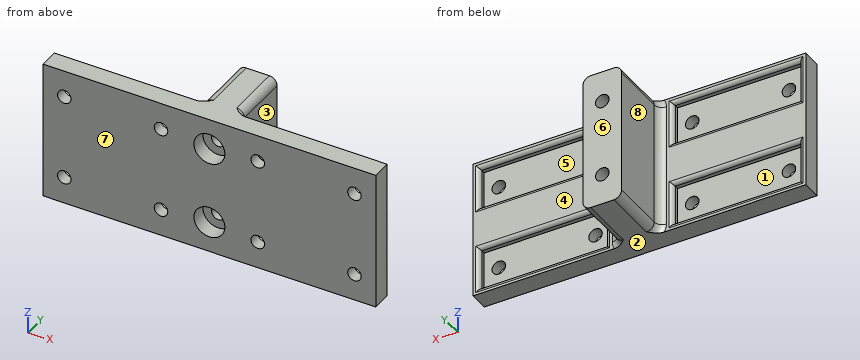
```python
from build123d import *

# Parameters (mm, degrees)
SKETCH_1_W          = 86
SKETCH_1_H          = 36
EXTRUDE_1_DEPTH     = 5
SKETCH_5_W          = 32.6
SKETCH_5_H          = 10.6
SKETCH_5_R          = 1.75
CUT_EXTRUDE_2_DEPTH = 2
SKETCH_5_3_R        = 1.75
CUT_EXTRUDE_3_DEPTH = 47.882832679
FILLET_2_R          = 1
SKETCH_8_W          = 10
SKETCH_8_H          = 36
EXTRUDE_2_DEPTH     = 16.5
SKETCH_9_R          = 1.75
CUT_EXTRUDE_4_DEPTH = 52.334686129
FILLET_3_R          = 2
FILLET_4_R          = 2
SKETCH_10_R         = 4
CUT_EXTRUDE_5_DEPTH = 4


with BuildPart() as part:
    # ｽｹｯﾁ1 → ﾎﾞｽ - 押し出し1 (new body)
    with BuildSketch(Plane(origin=(0, 0, 0), x_dir=(1, 0, 0), z_dir=(0, 1, 0))):
        Rectangle(SKETCH_1_W, SKETCH_1_H)
    extrude(amount=EXTRUDE_1_DEPTH)

    # ｽｹｯﾁ5 → ｶｯﾄ - 押し出し2 (cut)
    # profile 1 of 4: a face of its own
    with BuildSketch(Plane(origin=(0, 5, 0), x_dir=(1, 0, 0), z_dir=(0, 1, 0))):
        with Locations((-25, -11)):
            Rectangle(SKETCH_5_W, SKETCH_5_H)
        with Locations(Location((-37.5, -11, 0), (0, 0, 270))):
            Circle(SKETCH_5_R, mode=Mode.SUBTRACT)
        with Locations(Location((-12.5, -11, 0), (0, 0, 90))):
            Circle(SKETCH_5_R, mode=Mode.SUBTRACT)
    # profile 2 of 4: a face of its own
    with BuildSketch(Plane(origin=(0, 5, 0), x_dir=(1, 0, 0), z_dir=(0, 1, 0))):
        with Locations((-25, 11)):
            Rectangle(SKETCH_5_W, SKETCH_5_H)
        with Locations(Location((-12.5, 11, 0), (0, 0, 270))):
            Circle(SKETCH_5_R, mode=Mode.SUBTRACT)
        with Locations(Location((-37.5, 11, 0), (0, 0, 90))):
            Circle(SKETCH_5_R, mode=Mode.SUBTRACT)
    # profile 3 of 4: a face of its own
    with BuildSketch(Plane(origin=(0, 5, 0), x_dir=(1, 0, 0), z_dir=(0, 1, 0))):
        with Locations((25, 11)):
            Rectangle(SKETCH_5_W, SKETCH_5_H)
        with Locations(Location((37.5, 11, 0), (0, 0, 270))):
            Circle(SKETCH_5_R, mode=Mode.SUBTRACT)
        with Locations(Location((12.5, 11, 0), (0, 0, 90))):
            Circle(SKETCH_5_R, mode=Mode.SUBTRACT)
    # profile 4 of 4: a face of its own
    with BuildSketch(Plane(origin=(0, 5, 0), x_dir=(1, 0, 0), z_dir=(0, 1, 0))):
        with Locations((25, -11)):
            Rectangle(SKETCH_5_W, SKETCH_5_H)
        with Locations(Location((12.5, -11, 0), (0, 0, 270))):
            Circle(SKETCH_5_R, mode=Mode.SUBTRACT)
        with Locations(Location((37.5, -11, 0), (0, 0, 90))):
            Circle(SKETCH_5_R, mode=Mode.SUBTRACT)
    extrude(amount=-CUT_EXTRUDE_2_DEPTH, mode=Mode.SUBTRACT)

    # ｽｹｯﾁ5<3> → ｶｯﾄ - 押し出し3 (cut, through all)
    with BuildSketch(Plane(origin=(0, 5, 0), x_dir=(1, 0, 0), z_dir=(0, 1, 0))):
        with Locations(Location((37.5, -11, 0), (0, 0, 270))):
            Circle(SKETCH_5_3_R)
        with Locations(Location((12.5, -11, 0), (0, 0, 270))):
            Circle(SKETCH_5_3_R)
        with Locations(Location((37.5, 11, 0), (0, 0, 270))):
            Circle(SKETCH_5_3_R)
        with Locations(Location((12.5, 11, 0), (0, 0, 270))):
            Circle(SKETCH_5_3_R)
        with Locations(Location((-12.5, 11, 0), (0, 0, 270))):
            Circle(SKETCH_5_3_R)
        with Locations(Location((-12.5, -11, 0), (0, 0, 270))):
            Circle(SKETCH_5_3_R)
        with Locations(Location((-37.5, -11, 0), (0, 0, 270))):
            Circle(SKETCH_5_3_R)
        with Locations(Location((-37.5, 11, 0), (0, 0, 270))):
            Circle(SKETCH_5_3_R)
    extrude(amount=-CUT_EXTRUDE_3_DEPTH, mode=Mode.SUBTRACT)

    # ﾌｨﾚｯﾄ2
    fillet_2_edges = [part.edges().sort_by_distance(p)[0] for p in [
        (-8.7, 5, 11),
        (-25, 5, 5.7),
        (-41.3, 5, 11),
        (-25, 5, 16.3),
        (-25, 5, -16.3),
        (-41.3, 5, -11),
        (-25, 5, -5.7),
        (-8.7, 5, -11),
        (8.7, 5, -11),
        (25, 5, -5.7),
        (41.3, 5, -11),
        (25, 5, -16.3),
        (25, 5, 16.3),
        (41.3, 5, 11),
        (25, 5, 5.7),
        (8.7, 5, 11),
    ]]
    fillet(fillet_2_edges, radius=FILLET_2_R)

    # ｽｹｯﾁ8 → ﾎﾞｽ - 押し出し2 (add)
    with BuildSketch(Plane(origin=(0, 5, 0), x_dir=(1, 0, 0), z_dir=(0, 1, 0))):
        Rectangle(SKETCH_8_W, SKETCH_8_H)
    extrude(amount=EXTRUDE_2_DEPTH)

    # ｽｹｯﾁ9 → ｶｯﾄ - 押し出し4 (cut, through all)
    with BuildSketch(Plane(origin=(0, 21.5, 0), x_dir=(1, 0, 0), z_dir=(0, 1, 0))):
        with Locations(Location((0, -10, 0), (0, 0, 270))):
            Circle(SKETCH_9_R)
        with Locations(Location((0, 10, 0), (0, 0, 270))):
            Circle(SKETCH_9_R)
    extrude(amount=-CUT_EXTRUDE_4_DEPTH, mode=Mode.SUBTRACT)

    # ﾌｨﾚｯﾄ3
    fillet_3_edges = [part.edges().sort_by_distance(p)[0] for p in [
        (-5, 13.25, -18),
        (-5, 13.25, 18),
        (5, 13.25, 18),
        (5, 13.25, -18),
    ]]
    fillet(fillet_3_edges, radius=FILLET_3_R)

    # ﾌｨﾚｯﾄ4
    # the kernel refuses this fillet: 2 mm, written as the material it adds along each edge
    with BuildSketch(Plane(origin=(5, 5, 16), x_dir=(1, 0, 0), z_dir=(0, 0, -1)), Plane(origin=(-5, 5, -16), x_dir=(-1, 0, 0), z_dir=(0, 0, 1))) as fillet_4_piece_1:
        with BuildLine():
            CenterArc((FILLET_4_R, -FILLET_4_R), FILLET_4_R, 90, 90)
            Line((0, -FILLET_4_R), (0, 0))
            Line((0, 0), (FILLET_4_R, 0))
        make_face()
    extrude(amount=32)
    with BuildSketch(Plane(origin=(3, 5, 16), x_dir=(-0.5976672776328272, 0, -0.8017442392976484), z_dir=(0.8017442392976484, 0, -0.5976672776328272))) as fillet_4_piece_2_section:
        with BuildLine():
            CenterArc((2 + FILLET_4_R, FILLET_4_R), FILLET_4_R, 180, 90)
            Line((2 + FILLET_4_R, 0), (2, 0))
            Line((2, 0), (2, FILLET_4_R))
        make_face()
    fillet_4_piece_2 = revolve(axis=Axis((3, 5, 16), (0, 1, 0)), revolution_arc=233.296989237, mode=Mode.PRIVATE)
    fillet_4_piece_2 = split(fillet_4_piece_2, bisect_by=Plane(origin=(4.499877774, 5.623256904, 18), z_dir=(0, 0, -1)), keep=Keep.TOP, mode=Mode.PRIVATE)
    add(fillet_4_piece_2)
    with BuildSketch(Plane(origin=(-3, 5, 16), x_dir=(0.5976672776328272, 0, -0.8017442392976484), z_dir=(-0.8017442392976484, 0, -0.5976672776328272))) as fillet_4_piece_3_section:
        with BuildLine():
            CenterArc((2 + FILLET_4_R, -FILLET_4_R), FILLET_4_R, 90, 90)
            Line((2, -FILLET_4_R), (2, 0))
            Line((2, 0), (2 + FILLET_4_R, 0))
        make_face()
    fillet_4_piece_3 = revolve(axis=Axis((-3, 5, 16), (0, -1, 0)), revolution_arc=233.296989237, mode=Mode.PRIVATE)
    fillet_4_piece_3 = split(fillet_4_piece_3, bisect_by=Plane(origin=(-4.499877889, 5.623256622, 18), z_dir=(0, 0, -1)), keep=Keep.TOP, mode=Mode.PRIVATE)
    add(fillet_4_piece_3)
    with BuildSketch(Plane(origin=(-3, 5, -16), x_dir=(-1, 0, 0), z_dir=(0, 0, 1))) as fillet_4_piece_4_section:
        with BuildLine():
            CenterArc((2 + FILLET_4_R, -FILLET_4_R), FILLET_4_R, 90, 90)
            Line((2, -FILLET_4_R), (2, 0))
            Line((2, 0), (2 + FILLET_4_R, 0))
        make_face()
    fillet_4_piece_4 = revolve(axis=Axis((-3, 5, -16), (0, -1, 0)), revolution_arc=233.296989237, mode=Mode.PRIVATE)
    fillet_4_piece_4 = split(fillet_4_piece_4, bisect_by=Plane(origin=(-5.439550498, 5.334600403, -18), z_dir=(0, 0, 1)), keep=Keep.TOP, mode=Mode.PRIVATE)
    add(fillet_4_piece_4)
    with BuildSketch(Plane(origin=(3, 5, -16), x_dir=(-0.5976672776328279, 0, 0.8017442392976479), z_dir=(0.8017442392976479, 0, 0.5976672776328279))) as fillet_4_piece_5_section:
        with BuildLine():
            CenterArc((2 + FILLET_4_R, -FILLET_4_R), FILLET_4_R, 90, 90)
            Line((2, -FILLET_4_R), (2, 0))
            Line((2, 0), (2 + FILLET_4_R, 0))
        make_face()
    fillet_4_piece_5 = revolve(axis=Axis((3, 5, -16), (0, -1, 0)), revolution_arc=233.296989237, mode=Mode.PRIVATE)
    fillet_4_piece_5 = split(fillet_4_piece_5, bisect_by=Plane(origin=(4.499877909, 5.62325654, -18), z_dir=(0, 0, 1)), keep=Keep.TOP, mode=Mode.PRIVATE)
    add(fillet_4_piece_5)

    # ｽｹｯﾁ10 → ｶｯﾄ - 押し出し5 (cut)
    with BuildSketch(Plane(origin=(0, 0, 0), x_dir=(-1, 0, 0), z_dir=(0, -1, 0))):
        with Locations(Location((0, -10, 0), (0, 0, 90))):
            Circle(SKETCH_10_R)
        with Locations(Location((0, 10, 0), (0, 0, 90))):
            Circle(SKETCH_10_R)
    extrude(amount=-CUT_EXTRUDE_5_DEPTH, mode=Mode.SUBTRACT)


solid = part.part
```
Can you work these out from the model? Positions are in its coordinate system, mm. Face numbers are marked on the shaded views. A direction names the side the tool comes from. Round coordinates to 2 decimals unless told otherwise and drop trailing zeros. Loops run counter-clockwise (first coordinate to the right, second up) from the corner with the lowest first, then second, coordinate; pieces in that order, holes last. Notation, with made-up numbers: (50.25, 85.25) -> (68.25, 85.25) arc R18 cw to (68.25, 97.25) -> close; hole circle Ø7 at (23, 61.25). An arc over 180 degrees is marked (long way). Answer in a Markdown table with one row per item.
Item 1: If I drill on probe 1 along Z at (x, y) = (38.5, 3.5); probe 2 along X at (y, z) = (1, -11); probe 3 along X at (y, z) = (13.5, -6.5), over which ranges is the centre line in solid material (lowest first)?
Answer block:
| item | result |
|---|---|
| probe 1 | -18 to -16.3, -5.7 to 5.7, 16.3 to 18 |
| probe 2 | -43 to -39.25, -35.75 to -14.25, -10.75 to -3.87, 3.87 to 10.75, 14.25 to 35.75, 39.25 to 43 |
| probe 3 | -5 to 5 |
Item 2: Suppose I cut it at A-A, the plane x = -12.5. List the corners of the cut face in (y, z) for me, plus the area to 3 significant figures.
Answer block:
| item | result |
|---|---|
| outline | (0, -18) -> (5, -18) -> (5, -17.3) arc R1 ccw to (4, -16.3) -> (3, -16.3) -> (3, -12.75) -> (0, -12.75) -> close; (0, -9.25) -> (3, -9.25) -> (3, -5.7) -> (4, -5.7) arc R1 ccw to (5, -4.7) -> (5, 4.7) arc R1 ccw to (4, 5.7) -> (3, 5.7) -> (3, 9.25) -> (0, 9.25) -> close; (0, 12.75) -> (3, 12.75) -> (3, 16.3) -> (4, 16.3) arc R1 ccw to (5, 17.3) -> (5, 18) -> (0, 18) -> close |
| area | 116 mm² |
Item 3: Suppose I cut it at B-B, the plane y = 10.75. List the corners of the cut face in (x, z) for me.
Answer block:
| item | result |
|---|---|
| outline | (-5, -16) arc R2 ccw to (-3, -18) -> (3, -18) arc R2 ccw to (5, -16) -> (5, 16) arc R2 ccw to (3, 18) -> (-3, 18) arc R2 ccw to (-5, 16) -> close; hole circle Ø3.5 at (0, -10); hole circle Ø3.5 at (0, 10) |
Item 4: Suppose I cut it at D-D, the plane z = 10.5. Give the number of separate pieces and of enclosed holes in the cut face, plus the area to 3 significant figures.
Answer block:
| item | result |
|---|---|
| separate pieces | 6 |
| enclosed holes | 0 |
| area | 335 mm² |
Item 5: We'd pull the mould along Z, two halves only. Please class the marked faces 1, 2 and 3: released by +Z, released by -Z, zero draft, split by the parting line, or undercut.
Answer block:
| item | result |
|---|---|
| face 1 | undercut |
| face 2 | released by -Z |
| face 3 | zero draft |
Item 6: Will these pins go through, and if not, where does the flat tip stop? P1, Ø5, axis at x = 6, y = 12, coming from the -Z side; P2, Ø3, axis at x = -12.5, z = -11, coming from the +Y side; P3, Ø7, axis at y = 17, z = 0, coming from the +X side; P4, Ø5.5, axis at x = 29.5, z = 12.5, coming from the +Y side.
Answer block:
| item | result |
|---|---|
| P1 | z = -17.94 |
| P2 | through |
| P3 | x = 5 |
| P4 | y = 3 |
Item 7: Suppose I cut it at C-C, the plane z = -2. List the corners of the cut face in (x, y) for me.
Answer block:
| item | result |
|---|---|
| outline | (-43, 0) -> (43, 0) -> (43, 5) -> (7, 5) arc R2 cw to (5, 7) -> (5, 21.5) -> (-5, 21.5) -> (-5, 7) arc R2 cw to (-7, 5) -> (-43, 5) -> close |
Item 8: On a 3-axis mill with a long thin cutter (end or side, diameter ignored), from which of +Z, -Z, +X, -X, +Y, -Y can I reach the whole of each face in a straight line? I mean the marked faces 4, 5, 6, 7 and 8. Say none if no direction works.
Answer block:
| item | result |
|---|---|
| face 4 | +Z, -Z, +X, +Y |
| face 5 | +Y |
| face 6 | +Z, -Z, +X, -X, +Y |
| face 7 | +Z, -Z, +X, -X, -Y |
| face 8 | +Z, -Z, -X, +Y |
